Build history of the part. All positions in model axes, mm. Face numbers are marked on the shaded views. Round coordinates to 2 decimals unless told otherwise and drop trailing zeros. Loops run counter-clockwise (first coordinate to the right, second up) from the corner with the lowest first, then second, coordinate; pieces in that order, holes last. Notation, with made-up numbers: (-11, 83.5) - (4, 83.5) arc R13 cw to (4, 88.5) - close; hole circle Ø1 at (9, 72). An arc over 180 degrees is marked (long way). Use one line per item in the form item = value. Start each with the question number.
Q1. Saw through at C-C (y = 45). Give the cut face in (x, z).
Q2. Saw through at B-B (z = 0). Give the cut face in (x, y), then the cut area to 3 significant figures.
Q3. Saw through at D-D (y = 72.5). Give the cut face in (x, z).
Q4. Saw through at A-A (x = 0). Give the cut face in (y, z).
Q5. Drill centre lines: line 1 (Z direction, x = 0, y = 32); line 2 (Y direction, x = 11.75, z = 0); line 3 (Y direction, x = -8, z = -7). Where is each one in solid material? Low to high.
Q6. Mould opens along X. For the marked faces 1 and 2 say: released by +X, released by -X, zero draft, split by the parting line, or undercut.
Q7. Pin check, flat tips, straight feed: pin 1 (12 mm diameter, centred on x = 7.5, y = 34.5, fed in from -Z); pin 2 (1 mm diameter, centred on y = 77.5, z = -3, fed in from +X); pin 3 (10 mm diameter, centred on x = -6, y = 55.5, fed in from +Z); pin 4 (5 mm diameter, centred on x = 2, z = 6, fed in from -Y). Stop position of each tip, or through.
```python
from build123d import *

# Parameters (mm, degrees)
SKETCH2_R           = 12.5
SKETCH2_R_2         = 9.5
BOSS_EXTRUDE1_DEPTH = 90
SKETCH4_R           = 3
CUT_EXTRUDE1_DEPTH  = 10
SKETCH5_R           = 3
CUT_EXTRUDE2_DEPTH  = 10


with BuildPart() as part:
    # Sketch2 → Boss-Extrude1 (new body)
    with BuildSketch(Plane(origin=(0, 0, 0), x_dir=(1, 0, 0), z_dir=(0, 1, 0))):
        Circle(SKETCH2_R)
        Circle(SKETCH2_R_2, mode=Mode.SUBTRACT)
    extrude(amount=BOSS_EXTRUDE1_DEPTH)

    # Sketch4 → Cut-Extrude1 (cut)
    with BuildSketch(Plane(origin=(12.5, 0, 0), x_dir=(0, 0, -1), z_dir=(1, 0, 0))):
        with Locations((0, 60)):
            Circle(SKETCH4_R)
        with Locations((0, 45)):
            Circle(SKETCH4_R)
    extrude(amount=-CUT_EXTRUDE1_DEPTH, mode=Mode.SUBTRACT)

    # Sketch5 → Cut-Extrude2 (cut)
    with BuildSketch(Plane(origin=(-8.838834765, 0, -8.838834765), x_dir=(-0.707106781, 0, 0.707106781), z_dir=(-0.707106781, 0, -0.707106781))):
        with Locations((0, 60)):
            Circle(SKETCH5_R)
        with Locations((0, 45)):
            Circle(SKETCH5_R)
    cut_extrude2 = extrude(amount=-CUT_EXTRUDE2_DEPTH, mode=Mode.SUBTRACT)

    # Mirror1: Cut-Extrude2 across plane
    add(cut_extrude2.mirror(Plane.XY), mode=Mode.SUBTRACT)


solid = part.part
```
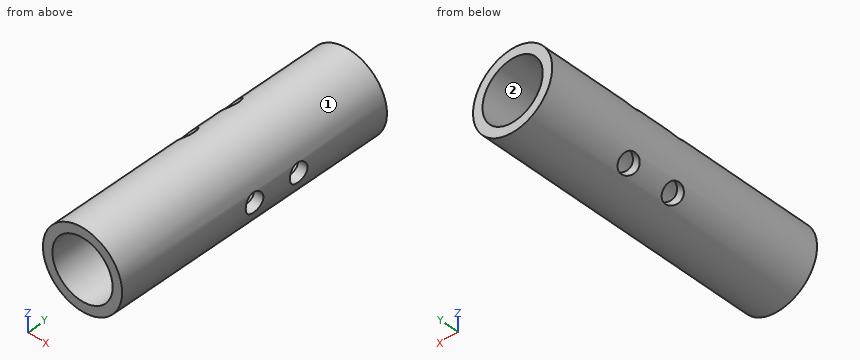
Report:
q1.outline = (-10.7, -6.46) - (-8.5, -4.25) arc R9.5 cw to (-8.5, 4.25) - (-10.7, 6.46) arc R12.5 ccw to start; (-6.46, -10.7) arc R12.5 ccw to (12.13, -3) - (9.01, -3) arc R9.5 cw to (-4.25, -8.5) - close; (-6.46, 10.7) - (-4.25, 8.5) arc R9.5 cw to (9.01, 3) - (12.13, 3) arc R12.5 ccw to start
q2.outline = (-12.5, 0) - (-9.5, 0) - (-9.5, 90) - (-12.5, 90) - close; (9.5, 0) - (12.5, 0) - (12.5, 42) - (9.5, 42) - close; (9.5, 48) - (12.5, 48) - (12.5, 57) - (9.5, 57) - close; (9.5, 63) - (12.5, 63) - (12.5, 90) - (9.5, 90) - close
q2.area = 504 mm²
q3.outline = circle Ø25 at (0, 0); hole circle Ø19 at (0, 0)
q4.outline = (0, -12.5) - (90, -12.5) - (90, -9.5) - (0, -9.5) - close; (0, 9.5) - (90, 9.5) - (90, 12.5) - (0, 12.5) - close
q5.line_1 = -12.5 to -9.5, 9.5 to 12.5
q5.line_2 = 0 to 42, 48 to 57, 63 to 90
q5.line_3 = 0 to 42.08, 47.92 to 57.08, 62.92 to 90
q6.face_1 = split by the parting line
q6.face_2 = undercut
q7.pin_1 = -12.41
q7.pin_2 = 12.25
q7.pin_3 = 12.46
q7.pin_4 = through
